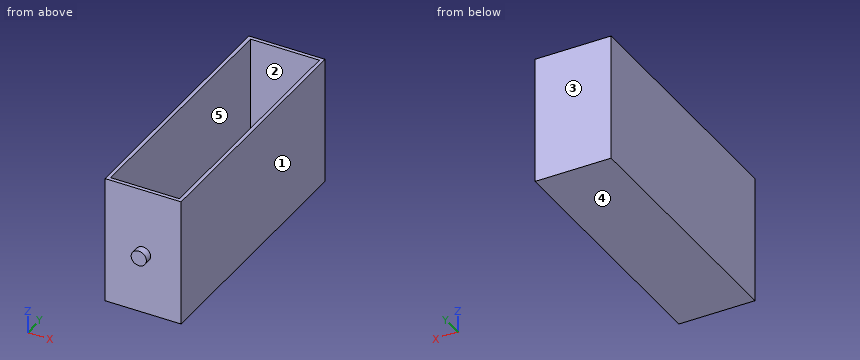
from build123d import *

# Parameters (mm, degrees)
F0_W     = 250
F0_H     = 850
F1_DEPTH = 12
F2_W     = 250
F2_H     = 850
F2_W_2   = 226
F2_H_2   = 826
F3_DEPTH = 408
F4_R     = 25
F5_DEPTH = 25


with BuildPart() as f1:
    # F0 (on Top) → F1 (new body)
    with BuildSketch(Plane.XY):
        with Locations((125, -425)):
            Rectangle(F0_W, F0_H)
    extrude(amount=F1_DEPTH)

    # F2 (on face) → F3 (join)
    with BuildSketch(Plane.XY.offset(12)):
        with Locations((125, -425)):
            Rectangle(F2_W, F2_H)
        with Locations((125, -425)):
            Rectangle(F2_W_2, F2_H_2, mode=Mode.SUBTRACT)
    extrude(amount=F3_DEPTH)

    # F4 (on face) → F5 (join)
    with BuildSketch(Plane.XZ.offset(850)):
        with Locations((125, 200)):
            Circle(F4_R)
    extrude(amount=F5_DEPTH)


solid = f1.part
Design review of the part built by this model. Coordinates are the model's own, in mm. Face numbers are marked on the shaded views. A direction names the side the tool comes from. Round coordinates to 2 decimals unless told otherwise and drop trailing zeros. Order: outer loops, then holes, each group sorted by start corner. A loop starts at its lowest first (then second) coordinate and runs counter-clockwise, first axis right, second up.
1) Draft analysis for pull direction Y (two halves, no side actions). For the marked faces 1, 2 and 3, state which applies: released by +Y, released by -Y, zero draft, split by the parting line, or undercut.
The answers:
face 1: zero draft
face 2: undercut
face 3: released by +Y
2) For L1, parallel to Y at x = 99, z = 200; L2, parallel to X at y = -178.5, z = 249; L3, parallel to Z at x = 192, y = -787, list the stretches that pass through material, from the lowest coordinate up.
The answers:
L1: y = -850 to -838, -12 to 0
L2: x = 0 to 12, 238 to 250
L3: z = 0 to 12
3) Consider section D-D (z = 200). State the section outline as (x, y) points, plus the area to 3 significant figures.
The answers:
outline: (0, -850) - (100, -850) - (100, -875) - (150, -875) - (150, -850) - (250, -850) - (250, 0) - (0, 0) - close; hole (12, -838) - (238, -838) - (238, -12) - (12, -12) - close
area: 27,100 mm2
4) Clearance check with flat-ended pins moving along their axes: pin 1 Ø2 at (x, z) = (131.5, 269.5) entering from -Y; pin 2 Ø6 at (x, y) = (30, -201.5) entering from +Z. State where each tip first meets the part, or that it passes through.
The answers:
pin 1: stops at y = -850
pin 2: stops at z = 12
5) Consider section A-A (z = 98.5). State the section outline as (x, y) points, plus the area to 3 significant figures.
The answers:
outline: (0, -850) - (250, -850) - (250, 0) - (0, 0) - close; hole (12, -838) - (238, -838) - (238, -12) - (12, -12) - close
area: 25,800 mm2
6) Consider section C-C (y = -757.5). State the section outline as (x, z) points, plus the area to 3 significant figures.
The answers:
outline: (0, 0) - (250, 0) - (250, 420) - (238, 420) - (238, 12) - (12, 12) - (12, 420) - (0, 420) - close
area: 12,800 mm2
7) Consider section B-B (x = 125). State the section outline as (y, z) points, plus the area to 3 significant figures.
The answers:
outline: (-875, 175) - (-850, 175) - (-850, 0) - (0, 0) - (0, 420) - (-12, 420) - (-12, 12) - (-838, 12) - (-838, 420) - (-850, 420) - (-850, 225) - (-875, 225) - close
area: 21,200 mm2
8) Machinability: for the marked faces 4 and 5, which of the approach directions +Z, -Z, +X, -X, +Y, -Y give a long, thin tool a straight path to every point of the face, cutting with its end or side? Answer none if there is none.
The answers:
face 4: -Z, +X, -X, +Y, -Y
face 5: +Z
